Autodesk Fusion 360 part; units mm, degrees
sketch "BoardFootprint" plane through (0, 0, 0) normal (0, 1, 0) x (1, 0, 0)
  line L0 (115, -30) -> (-115, -30)
  line L1 (-115, -30) -> (-115, 30)
  line L2 (-115, 30) -> (115, 30)
  line L3 (115, 30) -> (115, -30)
  line L4 (115, -30) -> (-115, 30) construction
  line L5 (-115, -30) -> (115, 30) construction
  circle A0 centre (-110, -25) radius 3
  circle A1 centre (-110, -25) radius 1.4
  circle A2 centre (110, -25) radius 3
  circle A3 centre (110, -25) radius 1.4
  circle A4 centre (-110, 25) radius 3
  circle A5 centre (-110, 25) radius 1.4
  circle A6 centre (110.2395, -0.0011) radius 3
  circle A7 centre (110.2395, -0.0011) radius 1.4
  dimension "d8" = 230
  dimension "d9" = 60
  dimension "d12" = 6
  dimension "d13" = 2.8
  dimension "d14" = 5
  dimension "d15" = 5
  dimension "d16" = 6
  dimension "d17" = 2.8
  dimension "d18" = 220
  dimension "d19" = 6
  dimension "d20" = 2.8
  dimension "d21" = 50
  dimension "d22" = 6
  dimension "d23" = 2.8
  dimension "d24" = 25
  dimension "d111" = 5
  dimension "d112" = 5
sketch "Frame" plane through (0, 0, 0) normal (0, 1, 0) x (1, 0, 0)
  circle A0 centre (-119, -25) radius 3
  circle A1 centre (-119, -25) radius 1.4
  circle A2 centre (-119, 25) radius 3
  circle A3 centre (-119, 25) radius 1.4
  line L0 (115, -30) -> (-115, -30)
  circle A4 centre (119, -25) radius 3
  circle A5 centre (119, -25) radius 1.4
  circle A6 centre (119, 25) radius 3
  circle A7 centre (119, 25) radius 1.4
  line L1 (-122, 28) -> (-116, 28) construction
  line L2 (-115, 30) -> (115, 30)
  line L3 (-124, 33.5) -> (124, 33.5)
  line L4 (124, 33.5) -> (124, -33.5)
  line L5 (124, -33.5) -> (-124, -33.5)
  line L6 (-124, -33.5) -> (-124, 33.5)
  line L7 (-122, 27.5) -> (-122, 22.5) construction
  line L8 (122, -22.5) -> (122, -27.5) construction
  line L9 (-121, 30.5) -> (121, 30.5)
  line L10 (121, 30.5) -> (121, -30.5)
  line L11 (121, -30.5) -> (-121, -30.5)
  line L12 (-121, -30.5) -> (-121, 30.5)
  point P0 (-110, -25)
  point P1 (-110, 25)
  point P2 (110, -25)
  dimension "d26" = 6
  dimension "d27" = 2.8
  dimension "d28" = 6
  dimension "d29" = 2.8
  dimension "d30" = 50
  dimension "d31" = 9
  dimension "d33" = 9
  dimension "d34" = 5
  dimension "d35" = 6
  dimension "d36" = 2.8
  dimension "d37" = 5
  dimension "d39" = 6
  dimension "d40" = 2.8
  dimension "d41" = 50
  dimension "d44" = 2
  dimension "d52" = 0.5
  dimension "d53" = 3
  dimension "d54" = 3
  dimension "d56" = 0.5
  dimension "d57" = 2
  dimension "d58" = 3
  dimension "d59" = 3
  dimension "d116" = 248
sketch "Interconnects" plane through (0, 0, 0) normal (0, 1, 0) x (1, 0, 0)
  line L0 (-117.6, 27) -> (-111.4, 27)
  line L1 (-111.4, 27) -> (-111.4, 23)
  line L2 (-111.4, 23) -> (-117.6, 23)
  line L3 (-117.6, 23) -> (-117.6, 27)
  circle A0 centre (-119, 25) radius 1.4
  circle A1 centre (-119, 25) radius 1.4
  circle A2 centre (-119, 25) radius 1.4
  circle A3 centre (-110, 25) radius 1.4
  line L4 (-117.6, -23) -> (-111.4, -23)
  line L5 (-111.4, -23) -> (-111.4, -27)
  line L6 (-111.4, -27) -> (-117.6, -27)
  line L7 (-117.6, -27) -> (-117.6, -23)
  line L8 (-120, -23) -> (-109, -23) construction
  line L9 (-120, -27) -> (-109, -27) construction
  circle A4 centre (-119, -25) radius 3
  circle A5 centre (-119, -25) radius 3
  circle A6 centre (-119, -25) radius 1.4
  circle A7 centre (-110, -25) radius 1.4
  circle A8 centre (-119, -25) radius 1.4
  circle A9 centre (-119, -25) radius 3
  circle A10 centre (-119, -25) radius 1.4
  line L10 (-119, 25) -> (-110, 25) construction
  line L11 (-119, -25) -> (-110, -25) construction
  line L12 (110, -25) -> (119, -25) construction
  line L13 (111.4, -23) -> (117.6, -23)
  line L14 (117.6, -23) -> (117.6, -27)
  line L15 (117.6, -27) -> (111.4, -27)
  line L16 (111.4, -27) -> (111.4, -23)
  circle A11 centre (119, -25) radius 1.4
  circle A12 centre (110, -25) radius 1.4
  line L17 (108.8395, 1.9989) -> (121, 1.9989)
  line L18 (121, 1.9989) -> (121, -2.0011)
  line L19 (121, -2.0011) -> (108.8395, -2.0011)
  line L20 (108.8395, -2.0011) -> (108.8395, 1.9989)
  line L21 (110.2395, -0.0011) -> (122, -0.0011) construction
  circle A13 centre (110.2395, -0.0011) radius 1.4
  line L22 (121, 30.5) -> (121, -30.5)
  point P0 (110, -25)
  point P1 (119, -25)
  point P2 (110.2395, -0.0011)
  dimension "d60" = 4
  dimension "d61" = 4
  dimension "d62" = 4
  dimension "d64" = 4
extrude "Extrude1" add sketch "BoardFootprint" sketch "Interconnects" against normal blind 16 contours A0 | A2 | A4 | A6 of sketch 2 contours L0 L1 L2 L3 | L4 L6 L7 A4 A5 A9 | L4 L5 L6 A4 A5 A9 | L13 L14 L15 L16 | A13 | L17 L18 L19 L20 L22 picked at (-117.2323, -26.2179) makes body 1 at (-108.8955, -10.6667, 27.7893) makes body 2 at (112.2704, -10.6667, 2.2092) makes body 3 at (-108.8955, -10.6667, -22.2107) makes body 4 at (112.0309, -10.6667, 27.2081)
extrude "Extrude2" add sketch "Frame" against normal blind 16 contours A0 L12 | A0 L12 | A2 L12 | A2 L12 | A4 L10 | A4 L10 | A6 L10 | A6 L10 | L3 L4 L5 L6 bodies 1 2 3 4
extrude "Extrude3" add sketch "Frame" along normal blind 16 contours A0 L12 | A0 L12 | A2 L12 | A2 L12 | A4 L10 | A4 L10 | A6 L10 | A6 L10 | L3 L4 L5 L6 bodies 1
extrude "Extrude4" cut sketch "Frame" against normal blind 18 contours A6 L10 picked at (120.8, 25) bodies 1
sketch "NanoMountR" plane through (121, 0, 0) normal (-1, 0, 0) x (0, 0, 1)
  line L0 (-1.9989, -16) -> (-1.9989, 0)
  line L1 (-1.9989, 0) -> (2.0011, 0)
  line L2 (2.0011, 0) -> (2.0011, -16)
  line L3 (2.0011, -16) -> (22.7639, -16)
  line L4 (22.7639, -16) -> (22.7639, 16)
  line L5 (22.7639, 16) -> (-22.7639, 16)
  line L6 (-22.7639, 16) -> (-22.7639, 0)
  line L7 (-22.7639, 0) -> (-27.2361, 0)
  line L8 (-27.2361, 0) -> (-27.2361, 16)
  line L9 (-27.2361, 16) -> (-30.5, 16)
  line L10 (-30.5, 16) -> (-30.5, -16)
  line L11 (-30.5, -16) -> (-1.9989, -16)
  line L12 (-30.5, -16) -> (-27.5, -16)
  line L13 (-27.5, -16) -> (-27.5, -13)
  line L14 (-27.5, -13) -> (-30.5, -13)
  line L15 (-30.5, -13) -> (-30.5, -16)
  line L16 (-15.5, -16) -> (-12.5, -16)
  line L17 (-15.5, -13) -> (-15.5, -16)
  line L18 (-12.5, -16) -> (-12.5, -13)
  line L19 (-12.5, -13) -> (-15.5, -13)
  point P0 (-15.5, -16)
  dimension "d73" = 3
  dimension "d74" = 3
  dimension "d75" = 3
  dimension "d76" = 3
  dimension "d77" = 12
extrude "Extrude5" add sketch "NanoMountR" along normal blind 3.2 contours L11 L16 L17 L18 L19 | L10 L11 L12 L13 L14 L15 bodies 1
sketch "NanoMountL" plane through (0, -13, 0) normal (0, 1, 0) x (-1, 0, 0)
  line L0 (-121, -27.5) -> (-121, -30.5)
  line L1 (-121, -30.5) -> (-117.8, -30.5)
  line L2 (-117.8, -30.5) -> (-117.8, -27.5)
  line L3 (-117.8, -27.5) -> (-121, -27.5)
  circle A0 centre (-119.4, -29) radius 0.5
  circle A1 centre (-119.4, -14) radius 0.5
  line L4 (-77, -30.5) -> (-80.2, -30.5)
  line L5 (-80.2, -30.5) -> (-80.2, -12.5)
  line L6 (-80.2, -12.5) -> (-77, -12.5)
  line L7 (-77, -12.5) -> (-77, -30.5)
  circle A2 centre (-78.6, -29) radius 0.5
  circle A3 centre (-78.6, -14) radius 0.5
  line L8 (121, -30.5) -> (-121, -30.5)
  line L9 (-121, -22.7639) -> (-121, 22.7639)
  line L10 (-117.8, -12.5) -> (-117.8, -15.5)
  line L11 (-121, -12.5) -> (-117.8, -12.5)
  point P0 (-121, -12.5)
  dimension "d80" = 1
  dimension "d81" = 1
  dimension "d82" = 15
  dimension "d83" = 1
  dimension "d84" = 1
  dimension "d85" = 15
  dimension "d98" = 1.5
  dimension "d99" = 1.5
  dimension "d100" = 40.8
  dimension "d101" = 1.6
  dimension "d102" = 37.6
extrude "Extrude6" add sketch "NanoMountL" against normal blind 3 contours L4 L5 L6 L7 L8 bodies 1
extrude "Extrude7" cut sketch "NanoMountL" against normal blind 3 contours A0 | A1 bodies 1
sketch "USBPort" plane through (121, 0, 0) normal (-1, 0, 0) x (0, 0, 1)
  line L0 (-15.5, -16) -> (-15.5, -13)
  line L1 (-15.5, -13) -> (-12.5, -13)
  line L2 (-12.5, -13) -> (-12.5, -16)
  line L3 (-12.5, -16) -> (-1.9989, -16)
  line L4 (-1.9989, -16) -> (-1.9989, 0)
  line L5 (-1.9989, 0) -> (2.0011, 0)
  line L6 (2.0011, 0) -> (2.0011, -16)
  line L7 (2.0011, -16) -> (22.7639, -16)
  line L8 (22.7639, -16) -> (22.7639, 16)
  line L9 (22.7639, 16) -> (-22.7639, 16)
  line L10 (-22.7639, 16) -> (-22.7639, 0)
  line L11 (-22.7639, 0) -> (-27.2361, 0)
  line L12 (-27.2361, 0) -> (-27.2361, 16)
  line L13 (-27.2361, 16) -> (-30.5, 16)
  line L14 (-30.5, 16) -> (-30.5, -13)
  line L15 (-30.5, -13) -> (-27.5, -13)
  line L16 (-27.5, -13) -> (-27.5, -16)
  line L17 (-27.5, -16) -> (-15.5, -16)
  line L18 (-26.5, -6.5) -> (-16.5, -6.5)
  line L19 (-16.5, -6.5) -> (-16.5, -12)
  line L20 (-16.5, -12) -> (-26.5, -12)
  line L21 (-26.5, -12) -> (-26.5, -6.5)
  line L22 (-12.5, -13) -> (-30.5, -13)
  line L23 (-21.5, -13) -> (-21.5, -5.5) construction
  dimension "d93" = 10
  dimension "d94" = 5.5
  dimension "d95" = 1
extrude "Extrude8" cut sketch "USBPort" against normal blind 4 contours L18 L19 L20 L21 bodies 1
sketch "Facia" plane through (0, 16, 0) normal (0, 1, 0) x (-1, 0, 0)
  circle A0 centre (-119, 25) radius 1.4
  circle A1 centre (119, 25) radius 1.4
  line L0 (-121, 30.5) -> (121, 30.5)
  line L1 (121, 30.5) -> (121, 27.2361)
  arc A2 (121, 27.2361) -> (121, 22.7639) centre (119, 25) ccw
  line L2 (121, 22.7639) -> (121, -22.7639)
  arc A3 (121, -22.7639) -> (121, -27.2361) centre (119, -25) ccw
  line L3 (121, -27.2361) -> (121, -30.5)
  line L4 (121, -30.5) -> (-121, -30.5)
  line L5 (-121, -30.5) -> (-121, -27.2361)
  arc A4 (-121, -27.2361) -> (-121, -22.7639) centre (-119, -25) ccw
  line L6 (-121, -22.7639) -> (-121, 22.7639)
  arc A5 (-121, 22.7639) -> (-121, 27.2361) centre (-119, 25) ccw
  line L7 (-121, 27.2361) -> (-121, 30.5)
  circle A6 centre (-119, -25) radius 1.4
  circle A7 centre (119, -25) radius 1.4
  line L8 (124, 33.5) -> (-124, 33.5)
  line L9 (-124, 33.5) -> (-124, -33.5)
  line L10 (-124, -33.5) -> (124, -33.5)
  line L11 (124, -33.5) -> (124, 33.5)
  line L12 (124.125, -33.625) -> (-124.125, -33.625)
  line L13 (-124.125, -33.625) -> (-124.125, 33.625)
  line L14 (-124.125, 33.625) -> (124.125, 33.625)
  line L15 (124.125, 33.625) -> (124.125, -33.625)
  line L16 (124, 33.5) -> (124, -33.5)
  line L17 (-124, -33.5) -> (-124, 33.5)
  line L18 (-124, 33.5) -> (124, 33.5)
  circle A8 centre (-119, 25) radius 1.9
  circle A9 centre (-119, -25) radius 1.9
  circle A10 centre (119, -25) radius 1.9
  circle A11 centre (119, 25) radius 1.9
  dimension "d103" = 0.125
  dimension "d104" = 0.125
  dimension "d105" = 0.125
  dimension "d106" = 0.125
  dimension "d107" = 3.8
  dimension "d108" = 3.8
  dimension "d109" = 3.8
  dimension "d110" = 3.8
extrude "Extrude9" cut sketch "BoardFootprint" against normal blind 61 contours A3 | A7 bodies 1
equation "VFDBoardWidth = 230 mm"
equation "VFDBoardHeight = 60 mm"
equation "LLPostVerticalOffset = 5 mm"
equation "LLPostHorizontalOffset = 5 mm"
equation "PostVerticalOffset1 = 50 mm"
equation "PostVerticalOffset2 = 25 mm"
equation "PostHorizontalOffset = 220 mm"
equation "d8 = VFDBoardWidth"
equation "d9 = VFDBoardHeight"
equation "PostInnerDiameter = 2.8 mm"
equation "PostOuterDiameter = 6 mm"
equation "d12 = PostOuterDiameter"
equation "d13 = PostInnerDiameter"
equation "d14 = LLPostVerticalOffset"
equation "d15 = LLPostHorizontalOffset"
equation "d16 = PostOuterDiameter"
equation "d17 = PostInnerDiameter"
equation "d18 = PostHorizontalOffset"
equation "d19 = PostOuterDiameter"
equation "d20 = PostInnerDiameter"
equation "d21 = PostVerticalOffset1"
equation "d22 = PostOuterDiameter"
equation "d23 = PostInnerDiameter"
equation "d24 = PostVerticalOffset2"
equation "d26 = PostOuterDiameter"
equation "d27 = PostInnerDiameter"
equation "d28 = PostOuterDiameter"
equation "d29 = PostInnerDiameter"
equation "d30 = PostVerticalOffset1"
equation "d31 = FaciaPostHorizontalOffset"
equation "FaciaPostHorizontalOffset = 9 mm"
equation "d33 = FaciaPostHorizontalOffset"
equation "d34 = LLPostVerticalOffset"
equation "d35 = PostOuterDiameter"
equation "d36 = PostInnerDiameter"
equation "d37 = LLPostVerticalOffset"
equation "d39 = PostOuterDiameter"
equation "d40 = PostInnerDiameter"
equation "d41 = PostVerticalOffset1"
equation "d44 = FramePostOffset"
equation "FrameThickness = 3 mm"
equation "FramePostOffset = 2 mm"
equation "FrameInnerSlop = 0.5 mm"
equation "d52 = FrameInnerSlop"
equation "d53 = FrameThickness"
equation "d54 = FrameThickness"
equation "d56 = FrameInnerSlop"
equation "d57 = FramePostOffset"
equation "d58 = FrameThickness"
equation "d59 = FrameThickness"
equation "d61 = InterconnectThickness"
equation "d62 = InterconnectThickness"
equation "InterconnectThickness = 4 mm"
equation "d64 = InterconnectThickness"
equation "USBPortWidth = 10 mm"
equation "USBPortHeight = 5.5 mm"
equation "USBPortVerticalOffset = 1 mm"
equation "d93 = USBPortWidth"
equation "d94 = USBPortHeight"
equation "d95 = USBPortVerticalOffset"
equation "d107 = PostInnerDiameter + 1.0 mm"
equation "d108 = PostInnerDiameter + 1 mm"
equation "d109 = PostInnerDiameter + 1 mm"
equation "d110 = PostInnerDiameter + 1 mm"
Design review of the part built by this model. Coordinates are the model's own, in mm. A direction names the side the tool comes from. Round coordinates to 2 decimals unless told otherwise and drop trailing zeros. Loops run counter-clockwise (first coordinate to the right, second up) from the corner with the lowest first, then second, coordinate; pieces in that order, holes last. Notation, with made-up numbers: (27.25, 84) -> (49.25, 84) arc R21 ccw to (49.25, 121) -> close; hole circle Ø1 at (45.25, 38). An arc over 180 degrees is marked (long way). Use one line per item in the form item = value. Start each with the question number.
Q1. We need section D-D on y = -9. State how many separate pieces and enclosed holes the cut face has, then the cut area to 3 significant figures.
Q2. Machinability: for faces 4 (the face through (124, 0, 0)), 5 (the face through (114, 0, 0)), 6 (the face through (-115, -8, -27)), which of the approach directions +Z, -Z, +X, -X, +Y, -Y give a long, thin tool a straight path to every point of the face, cutting with its end or side? Answer none if there is none.
Q3. For pin 1 Ø1.5 at (x, z) = (118.5, -29.5) entering from +Y; pin 2 Ø2.5 at (x, z) = (118.5, -24) entering from -Y, all flat-tipped, find the tip position at first contact; note any pin that passes through.
Q4. Draft analysis for pull direction Z (two halves, no side actions). For faces 1 (the face through (-116, 0.2, -24.9)), 2 (the face through (-124, 0, 0)), 3 (the face through (2, 0, 33.5)), state which applies: +Z half, -Z half, draft (parallel to the pull), parting line (faces both ways), or undercut.
Q5. We need section A-A on z = 9. Give the boundary of the cut face in (x, y), then the cut area to 3 significant figures.
Q6. We need section B-B on x = -99. Give the boundary of the cut face in (y, z), then the cut area to 3 significant figures.
Q7. Wall thickness on line 1 along Z through (x, y) = (-110, -3.5); line 2 along X through (y, z) = (-2.5, 25); line 3 along Z through (x, y) = (110, -5.75): over which ranges is each line inside the solid? List them lowest first. Write a range as [from, to].
Q8. We need section C-C on y = 6.5. Give the boundary of the cut face in (x, z).
Calculated:
q1.separate_pieces = 1
q1.enclosed_holes = 7
q1.area = 2,040 mm²
q2.face_4 = +Z, -Z, +X, +Y, -Y
q2.face_5 = +Y
q2.face_6 = +Y, -Y
q3.pin_1 = -13
q3.pin_2 = 0
q4.face_1 = undercut
q4.face_2 = draft
q4.face_3 = +Z half
q5.outline = (-124, -16) -> (-121, -16) -> (-121, 16) -> (-124, 16) -> close; (121, -16) -> (124, -16) -> (124, 16) -> (121, 16) -> close
q5.area = 192 mm²
q6.outline = (-16, -33.5) -> (16, -33.5) -> (16, -30.5) -> (-16, -30.5) -> close; (-16, 30.5) -> (16, 30.5) -> (16, 33.5) -> (-16, 33.5) -> close
q6.area = 192 mm²
q7.line_1 = [-33.5, -30.5], [-28, -26.4], [-23.6, -22], [22, 23.6], [26.4, 28], [30.5, 33.5]
q7.line_2 = [-124, -120.4], [-117.6, -111.4], [-108.6, -107], [107, 108.6], [111.4, 117.6], [120.4, 124]
q7.line_3 = [-33.5, -30.5], [-2.99, -1.38], [1.38, 2.99], [22, 23.6], [26.4, 28], [30.5, 33.5]
q8.outline = (-124, -33.5) -> (124, -33.5) -> (124, 33.5) -> (-124, 33.5) -> close; hole (-121, -30.5) -> (121, -30.5) -> (121, -27.24) arc R3 cw (long way) to (121, -22.76) -> (121, 22.76) arc R3 cw (long way) to (121, 27.24) -> (121, 30.5) -> (-121, 30.5) -> (-121, 27.24) arc R3 cw (long way) to (-121, 22.76) -> (-121, -22.76) arc R3 cw (long way) to (-121, -27.24) -> close; hole circle Ø2.8 at (-119, -25); hole circle Ø2.8 at (-119, 25); hole circle Ø2.8 at (119, -25); hole circle Ø2.8 at (119, 25)
